```python
from build123d import *

# Parameters (mm, degrees)
BOSS_EXTRUDE1_DEPTH               = 1.8415
SKETCH2_R                         = 3.8989
BOSS_EXTRUDE2_DEPTH               = 1.27
F_1_4_20_TAPPED_HOLE1_D           = 5.1054
F_1_4_20_TAPPED_HOLE1_DEPTH       = 16.51
F_1_4_20_TAPPED_HOLE1_CBORE_D     = 6.35
F_1_4_20_TAPPED_HOLE1_CBORE_DEPTH = 12.7
F_1_4_20_TAPPED_HOLE1_TIP         = 1.533816902


with BuildPart() as part:
    # Sketch1 → Boss-Extrude1 (new, symmetric)
    with BuildSketch(Plane.XY):
        with BuildLine():
            Line((-31.017747277, 8.3185), (31.017747277, 8.3185))
            ThreePointArc((31.017747277, 8.3185), (35.9029, 0), (31.017747277, -8.3185))
            Line((31.017747277, -8.3185), (-31.017747277, -8.3185))
            ThreePointArc((-31.017747277, -8.3185), (-35.9029, 0), (-31.017747277, 8.3185))
        make_face()
    extrude(amount=BOSS_EXTRUDE1_DEPTH, both=True)

    # Sketch2 → Boss-Extrude2 (add)
    with BuildSketch(Plane.XY.offset(1.8415)):
        with Locations((19.05, 0)):
            Circle(SKETCH2_R)
        with Locations((-19.05, 0)):
            Circle(SKETCH2_R)
    extrude(amount=BOSS_EXTRUDE2_DEPTH)

    # 1/4-20 Tapped Hole1
    with Locations(Plane(origin=(0, 0, -1.8415), x_dir=(-1, 0, 0), z_dir=(0, 0, -1))):
        with Locations((19.05, 0), (-19.05, 0)):
            CounterBoreHole(F_1_4_20_TAPPED_HOLE1_D / 2, F_1_4_20_TAPPED_HOLE1_CBORE_D / 2, F_1_4_20_TAPPED_HOLE1_CBORE_DEPTH, depth=F_1_4_20_TAPPED_HOLE1_DEPTH)
            with Locations((0, 0, -(F_1_4_20_TAPPED_HOLE1_DEPTH + F_1_4_20_TAPPED_HOLE1_TIP / 2))):  # 118° drill point
                Cone(0, F_1_4_20_TAPPED_HOLE1_D / 2, F_1_4_20_TAPPED_HOLE1_TIP, mode=Mode.SUBTRACT)


solid = part.part
```
Can you work these out from the model? Positions are in its coordinate system, mm. A direction names the side the tool comes from. Give positions to 0.01 mm unless a question says otherwise; leave off trailing zeros. Loops run counter-clockwise (first coordinate to the right, second up) from the corner with the lowest first, then second, coordinate; pieces in that order, holes last. Notation, with made-up numbers: M 54,14 L 66,14 A17 ccw 66,29 Z; hole C 53,26.25 d10. An arc over 180 degrees is marked long. Answer in a Markdown table with one row per item.
1. For pin 1 Ø2 at (y, z) = (-4, 2.5) entering from +X, with a flat end and sliding along its axis, tell me the tip position at first contact or that it passes through.
Taken from the geometry:
| item | result |
|---|---|
| pin 1 | stops at x = 35.33 |
2. Suppose I cut it at B-B on x = -19.05. Write out the boundary of the cut face in (y, z) (1 decimal), plus the area to 3 significant figures.
Taken from the geometry:
| item | result |
|---|---|
| outline | M -8.3,-1.8 L -3.2,-1.8 L -3.2,3.1 L -3.9,3.1 L -3.9,1.8 L -8.3,1.8 Z; M 3.2,-1.8 L 8.3,-1.8 L 8.3,1.8 L 3.9,1.8 L 3.9,3.1 L 3.2,3.1 Z |
| area | 39.7 mm² |
3. Suppose I cut it at C-C on z = 1.15. Count the separate pieces of the cut face and the enclosed holes in it, plus the area to 3 significant figures.
Taken from the geometry:
| item | result |
|---|---|
| separate pieces | 1 |
| enclosed holes | 2 |
| area | 1,080 mm² |
4. If I drill on line 1 along Y through (x, z) = (-19.05, -0.1) (1 decimal); line 2 along Z through (x, y) = (-33, -1.25); line 3 along X through (y, z) = (-2.5, 2.3), over which ranges is the centre line in solid material (lowest first)?
Taken from the geometry:
| item | result |
|---|---|
| line 1 | y = -8.3 to -3.2, 3.2 to 8.3 |
| line 2 | z = -1.84 to 1.84 |
| line 3 | x = -22.04 to -21.01, -17.09 to -16.06, 16.06 to 17.09, 21.01 to 22.04 |
5. Which directions (+Z, -Z, +X, -X, +Y, -Y) give clear straight access to the entire face, cutting with the end or side of a thin tool? Please do faces 4 (the cylindrical face through (-35.9, -0.14, 0.03)), 5 (the cylindrical face through (-22.945, 0.171, 2.468)).
Taken from the geometry:
| item | result |
|---|---|
| face 4 | +Z, -Z, -X |
| face 5 | +Z |
6. Suppose I cut it at D-D on x = 6. Write out the boundary of the cut face in (y, z), plus the area to 3 significant figures.
Taken from the geometry:
| item | result |
|---|---|
| outline | M -8.32,-1.84 L 8.32,-1.84 L 8.32,1.84 L -8.32,1.84 Z |
| area | 61.3 mm² |
7. Suppose I cut it at A-A on y = 0. Write out the boundary of the cut face in (x, z) (1 decimal).
Taken from the geometry:
| item | result |
|---|---|
| outline | M -35.9,-1.8 L -22.2,-1.8 L -22.2,3.1 L -22.9,3.1 L -22.9,1.8 L -35.9,1.8 Z; M -15.9,-1.8 L 15.9,-1.8 L 15.9,3.1 L 15.2,3.1 L 15.2,1.8 L -15.2,1.8 L -15.2,3.1 L -15.9,3.1 Z; M 22.2,-1.8 L 35.9,-1.8 L 35.9,1.8 L 22.9,1.8 L 22.9,3.1 L 22.2,3.1 Z |
8. Thinking about a two-plate mould opening in X: for faces 1 (the flat face through (0, -8.318, 0)), 2 (the cylindrical face through (-15.88, 0.14, 0.6)), 3 (the cylindrical face through (35.9, 0.14, 0.03)), which applies, released by +X, released by -X, zero draft, split by the parting line, or undercut?
Taken from the geometry:
| item | result |
|---|---|
| face 1 | zero draft |
| face 2 | undercut |
| face 3 | released by +X |
